Autodesk Inventor part; units mm, degrees
sketch "Sketch1" plane through (0, 0, 0) normal (0, 0, 1) x (1, 0, 0)
  line L0 (0, 2.8582) -> (0, -2.8582) construction
  line L1 (-5.7775, 0) -> (5.7775, 0) construction
  line L2 (-165, -75) -> (165, -75)
  line L3 (165, -75) -> (165, 75)
  line L4 (165, 75) -> (-165, 75)
  line L5 (-165, 75) -> (-165, -75)
  line L6 (-165, -75) -> (165, 75) construction
  line L7 (165, -75) -> (-165, 75) construction
  point P0 (0, 0)
  point P1 (0, 0)
  dimension "d0" = 330
  dimension "d1" = 150
extrude "Extrusion1" add sketch "Sketch1" along normal blind 5
sketch "Sketch2" plane through (0, 0, 5) normal (0, 0, 1) x (1, 0, 0)
  line L0 (0, 0) -> (-130, 0)
  circle A0 centre (-130, 0) radius 5
  line L1 (-165, 75) -> (-165, -75)
  line L2 (-165, 0) -> (-165, 15)
  line L3 (-165, 15) -> (-165, -15)
  line L4 (-165, -15) -> (-165, -45)
  line L5 (-165, -45) -> (-165, -75)
  line L6 (-165, 15) -> (-165, 45)
  line L7 (-165, 45) -> (-165, 75)
  line L8 (-165, 15) -> (-160, 15)
  line L9 (-160, 15) -> (-160, 45)
  line L10 (-160, 45) -> (-165, 45)
  line L11 (-165, 45) -> (-165, 15)
  line L12 (-165, -15) -> (-160, -15)
  line L13 (-160, -15) -> (-160, -45)
  line L14 (-160, -45) -> (-165, -45)
  line L15 (-165, -45) -> (-165, -15)
  line L16 (-165, -75) -> (165, -75)
  line L17 (-165, -75) -> (-135, -75)
  line L18 (-135, -75) -> (-105, -75)
  line L19 (-105, -75) -> (-75, -75)
  line L20 (-75, -75) -> (-45, -75)
  line L21 (-45, -75) -> (-15, -75)
  line L22 (-15, -75) -> (15, -75)
  line L23 (15, -75) -> (45, -75)
  line L24 (45, -75) -> (75, -75)
  line L25 (75, -75) -> (105, -75)
  line L26 (105, -75) -> (135, -75)
  line L27 (135, -75) -> (165, -75)
  line L28 (-165, -75) -> (-135, -75)
  line L29 (-135, -75) -> (-135, -70)
  line L30 (-135, -70) -> (-165, -70)
  line L31 (-165, -70) -> (-165, -75)
  line L32 (-105, -75) -> (-75, -75)
  line L33 (-75, -75) -> (-75, -70)
  line L34 (-75, -70) -> (-105, -70)
  line L35 (-105, -70) -> (-105, -75)
  line L36 (-45, -75) -> (-15, -75)
  line L37 (-15, -75) -> (-15, -70)
  line L38 (-15, -70) -> (-45, -70)
  line L39 (-45, -70) -> (-45, -75)
  line L40 (15, -75) -> (45, -75)
  line L41 (45, -75) -> (45, -70)
  line L42 (45, -70) -> (15, -70)
  line L43 (15, -70) -> (15, -75)
  line L44 (75, -75) -> (105, -75)
  line L45 (105, -75) -> (105, -70)
  line L46 (105, -70) -> (75, -70)
  line L47 (75, -70) -> (75, -75)
  line L48 (135, -75) -> (165, -75)
  line L49 (165, -75) -> (165, -70)
  line L50 (165, -70) -> (135, -70)
  line L51 (135, -70) -> (135, -75)
  line L52 (165, 75) -> (-165, 75)
  line L53 (-165, 75) -> (-135, 75)
  line L54 (-135, 75) -> (-135, 70)
  line L55 (-135, 70) -> (-165, 70)
  line L56 (-165, 70) -> (-165, 75)
  line L57 (-105, 75) -> (-75, 75)
  line L58 (-75, 75) -> (-75, 70)
  line L59 (-75, 70) -> (-105, 70)
  line L60 (-105, 70) -> (-105, 75)
  line L61 (-45, 75) -> (-15, 75)
  line L62 (-15, 75) -> (-15, 70)
  line L63 (-15, 70) -> (-45, 70)
  line L64 (-45, 70) -> (-45, 75)
  line L65 (15, 75) -> (45, 75)
  line L66 (45, 75) -> (45, 70)
  line L67 (45, 70) -> (15, 70)
  line L68 (15, 70) -> (15, 75)
  line L69 (75, 75) -> (105, 75)
  line L70 (105, 75) -> (105, 70)
  line L71 (105, 70) -> (75, 70)
  line L72 (75, 70) -> (75, 75)
  line L73 (165, -75) -> (165, 75)
  line L74 (135, 75) -> (165, 75)
  line L75 (165, 75) -> (165, 70)
  line L76 (165, 70) -> (135, 70)
  line L77 (135, 70) -> (135, 75)
  line L78 (165, 0) -> (165, 15)
  line L79 (165, 15) -> (160, 15)
  line L80 (160, 15) -> (160, 45)
  line L81 (160, 45) -> (165, 45)
  line L82 (165, 45) -> (165, 15)
  line L83 (165, -15) -> (160, -15)
  line L84 (160, -15) -> (160, -45)
  line L85 (160, -45) -> (165, -45)
  line L86 (165, -45) -> (165, -15)
  point P0 (-165, -70)
  point P1 (135, 75)
  point P2 (105, 75)
  point P3 (75, 75)
  point P4 (45, 75)
  point P5 (15, 75)
  point P6 (-15, 75)
  point P7 (-165, 70)
  point P8 (-165, -45)
  dimension "d4" = 130
  dimension "d5" = 10
  dimension "d6" = 15
  dimension "d7" = 30
  dimension "d8" = 30
  dimension "d9" = 30
  dimension "d10" = 30
  dimension "d11" = 30
  dimension "d12" = 5
  dimension "d13" = 30
  dimension "d14" = 30
  dimension "d15" = 30
  dimension "d16" = 30
  dimension "d17" = 30
  dimension "d18" = 30
  dimension "d19" = 30
  dimension "d20" = 30
  dimension "d21" = 30
  dimension "d22" = 30
  dimension "d23" = 30
  dimension "d24" = 5
  dimension "d25" = 5
  dimension "d26" = 5
  dimension "d29" = 30
  dimension "d30" = 30
  dimension "d31" = 30
  dimension "d32" = 30
  dimension "d33" = 30
  dimension "d34" = 30
extrude "Extrusion2" cut sketch "Sketch2" against normal blind 5 contours A0 | L52 L54 L55 L1 | L10 L9 L8 L1 | L52 L58 L59 L60 | L52 L62 L63 L64 | L12 L13 L14 L1 | L52 L66 L67 L68 | L30 L29 L16 L1 | L52 L70 L71 L72 | L35 L34 L33 L16 | L52 L73 L76 L77 | L39 L38 L37 L16 | L73 L79 L80 L81 | L43 L42 L41 L16 | L47 L46 L45 L16 | L73 L85 L84 L83 | L51 L50 L49 L16
sketch "Sketch3" plane through (0, 0, 5) normal (0, 0, 1) x (1, 0, 0)
  line L0 (165, -15) -> (165, 15)
  line L1 (165, 0) -> (85, 0)
  circle A0 centre (85, 0) radius 33.5
  point P0 (0, 0)
  dimension "d35" = 80
  dimension "d36" = 67
extrude "Extrusion3" cut sketch "Sketch3" against normal blind 10
sketch "Sketch4" plane through (0, 0, 5) normal (0, 0, 1) x (1, 0, 0)
  circle A0 centre (85, 0) radius 33.5
  line L0 (85, 0) -> (85, 42)
  circle A1 centre (85, 42) radius 2.5
  line L1 (85, 0) -> (85, -42)
  circle A2 centre (85, -42) radius 2.5
  point P0 (0, 0)
  dimension "d39" = 42
  dimension "d40" = 5
  dimension "d41" = 42
  dimension "d42" = 5
extrude "Extrusion4" cut sketch "Sketch4" against normal blind 5 contours A2 | A1
sketch "Sketch5" plane through (0, 0, 5) normal (0, 0, 1) x (1, 0, 0)
  line L0 (165, -70) -> (165, -45)
  line L1 (165, -70) -> (-75, -70)
  line L2 (-75, -70) -> (-75, 78.5235)
  line L3 (-75, 78.5235) -> (165, 78.5235)
  line L4 (165, 78.5235) -> (165, -70)
  line L5 (-75, 78.5235) -> (-190.1634, 78.5235)
  line L6 (-190.1634, 78.5235) -> (-190.1634, -89.7899)
  line L7 (-190.1634, -89.7899) -> (-75, -89.7899)
  line L8 (-75, -89.7899) -> (-75, 78.5235)
  point P0 (0, 0)
  dimension "d45" = 240
extrude "Extrusion5" cut sketch "Sketch5" against normal blind 10 contours L8 L7 L6 L5 L2
properties part number "Plaat boven" material "S235"
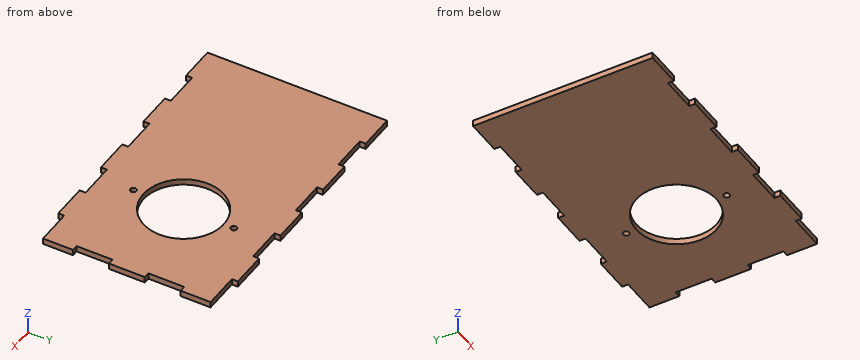
Input: part model. Units: mm. Frame: model coordinates. Coordinates: 2 decimals unless noted, no trailing zeros. Order: outer loops, then holes, each group sorted by start corner. A loop starts at its lowest first (then second) coordinate and runs counter-clockwise, first axis right, second up. Notation, with made-up numbers: (23.25, 23.25) - (68.25, 23.25) arc R25 ccw to (68.25, 56.25) - close; hole circle Ø2 at (18.5, -40). An arc over 180 degrees is marked (long way). Return JSON: item names as keys, results as strings.
Q1. Cut plane A-A (y = 0). Return loops of the section in (x, z), then the cut area to 3 significant figures.
The answers:
{"outline": "(-75, 0) - (51.5, 0) - (51.5, 5) - (-75, 5) - close; (118.5, 0) - (165, 0) - (165, 5) - (118.5, 5) - close", "area": "865 mm2"}
Q2. Cut plane C-C (y = 42). Return loops of the section in (x, z), then the cut area to 3 significant figures.
The answers:
{"outline": "(-75, 0) - (82.5, 0) - (82.5, 5) - (-75, 5) - close; (87.5, 0) - (160, 0) - (160, 5) - (87.5, 5) - close", "area": "1,150 mm2"}
Q3. Cut plane D-D (z = 2). State how many separate pieces and enclosed holes the cut face has, then the cut area to 3 significant figures.
The answers:
{"separate pieces": "1", "enclosed holes": "3", "area": "30,900 mm2"}
Q4. Ray query, probe 1 along Y at (x, z) = (85, 1.4); probe 2 along X at (y, z) = (-42, 1.55); probe 3 along X at (y, z) = (39, 2.7). Return the intervals inside material, ascending.
The answers:
{"probe 1": "y = -70 to -44.5, -39.5 to -33.5, 33.5 to 39.5, 44.5 to 70", "probe 2": "x = -75 to 82.5, 87.5 to 160", "probe 3": "x = -75 to 160"}
Q5. First-contact query: pin 1 (1.5 mm diameter, centred on y = -72, z = 2.5, fed in from +X); pin 2 (2.5 mm diameter, centred on x = 30.5, z = 2, fed in from -Y); pin 3 (1.5 mm diameter, centred on x = 40.5, z = 1.5, fed in from +Y). Flat tips, straight axial feed; report the tip coordinate or a pass-through.
The answers:
{"pin 1": "stops at x = 135", "pin 2": "stops at y = -70", "pin 3": "stops at y = 70"}
Q6. Cut plane B-B (x = 85). Return loops of the section in (y, z), then the cut area to 3 significant figures.
The answers:
{"outline": "(-70, 0) - (-44.5, 0) - (-44.5, 5) - (-70, 5) - close; (-39.5, 0) - (-33.5, 0) - (-33.5, 5) - (-39.5, 5) - close; (33.5, 0) - (39.5, 0) - (39.5, 5) - (33.5, 5) - close; (44.5, 0) - (70, 0) - (70, 5) - (44.5, 5) - close", "area": "315 mm2"}
